from build123d import *

# Parameters (mm, degrees)
AUFSATZ_LINEAR_AUSTRAGEN1_DEPTH = 24
VERRUNDUNG1_R                   = 2
SKIZZE6_R                       = 2.3
SCHNITT_LINEAR_AUSTRAGEN2_DEPTH = 100
SKIZZE7_W                       = 12.2
SKIZZE7_H                       = 11.3
SCHNITT_LINEAR_AUSTRAGEN3_DEPTH = 56.3
SCHNITT_LINEAR_AUSTRAGEN4_DEPTH = 25
SCHNITT_LINEAR_AUSTRAGEN5_DEPTH = 13.7
VERRUNDUNG2_R                   = 2
SCHNITT_LINEAR_AUSTRAGEN6_DEPTH = 23.5


with BuildPart() as part:
    # Skizze1 → Aufsatz-Linear austragen1 (new body)
    with BuildSketch(Plane(origin=(0, 0, 0), x_dir=(1, 0, 0), z_dir=(0, 1, 0))):
        with BuildLine():
            Line((-29.15, 22), (-29.15, 0))
            Line((-29.15, 0), (-21.15, 0))
            ThreePointArc((-21.15, 0), (-17.325065737, 12.131141629), (-7.233726031, 19.87449893))
            ThreePointArc((-7.233726031, 19.87449893), (-3.065111361, 19.529851295), (-0.617075906, 16.138206757))
            ThreePointArc((-0.617075906, 16.138206757), (11.199480437, 11.635898674), (16.15, 0))
            Line((16.15, 0), (26.15, 0))
            Line((26.15, 0), (26.15, 22.8))
            Line((26.15, 22.8), (17.65, 22.8))
            Line((17.65, 22.8), (17.65, 35))
            Line((17.65, 35), (-17.45, 35))
            Line((-17.45, 35), (-17.45, 22))
            Line((-17.45, 22), (-29.15, 22))
        make_face()
    extrude(amount=AUFSATZ_LINEAR_AUSTRAGEN1_DEPTH)

    # Verrundung1
    verrundung1_edges = [part.edges().sort_by_distance(p)[0] for p in [
        (-17.45, 12, -22),
    ]]
    fillet(verrundung1_edges, radius=VERRUNDUNG1_R)

    # Skizze6 → Schnitt-Linear austragen2 (cut)
    with BuildSketch(Plane.XY):
        with Locations((-24.15, 19)):
            Circle(SKIZZE6_R)
        with Locations((-24.15, 5)):
            Circle(SKIZZE6_R)
        with BuildLine():
            Line((-25.3, 17.008141571), (-24.15, 16.344188762))
            Line((-24.15, 16.344188762), (-23, 17.008141571))
            ThreePointArc((-23, 17.008141571), (-24.15, 16.7), (-25.3, 17.008141571))
        make_face()
        with BuildLine():
            Line((-25.3, 3.008141571), (-24.15, 2.344188762))
            Line((-24.15, 2.344188762), (-23, 3.008141571))
            ThreePointArc((-23, 3.008141571), (-24.15, 2.7), (-25.3, 3.008141571))
        make_face()
    extrude(amount=-SCHNITT_LINEAR_AUSTRAGEN2_DEPTH, mode=Mode.SUBTRACT)

    # Skizze7 → Schnitt-Linear austragen3 (cut, through all)
    with BuildSketch(Plane(origin=(26.15, 0, 0), x_dir=(0, 0, -1), z_dir=(1, 0, 0))):
        with Locations((28.9, 5.65)):
            Rectangle(SKIZZE7_W, SKIZZE7_H)
    extrude(amount=-SCHNITT_LINEAR_AUSTRAGEN3_DEPTH, mode=Mode.SUBTRACT)

    # Skizze8 → Schnitt-Linear austragen4 (cut)
    with BuildSketch(Plane(origin=(0, 0, -22.8), x_dir=(-1, 0, 0), z_dir=(0, 0, -1))):
        with BuildLine():
            Line((-22.275, 3.551442841), (-21.15, 2.901923789))
            Line((-21.15, 2.901923789), (-20.025, 3.551442841))
            ThreePointArc((-20.025, 3.551442841), (-21.15, 7.75), (-22.275, 3.551442841))
        make_face()
        with BuildLine():
            Line((-22.275, 17.051442841), (-21.15, 16.401923789))
            Line((-21.15, 16.401923789), (-20.025, 17.051442841))
            ThreePointArc((-20.025, 17.051442841), (-21.15, 21.25), (-22.275, 17.051442841))
        make_face()
    extrude(amount=-SCHNITT_LINEAR_AUSTRAGEN4_DEPTH, mode=Mode.SUBTRACT)

    # Skizze10 → Schnitt-Linear austragen5 (cut, through all)
    with BuildSketch(Plane.XZ.offset(-11.3)):
        with BuildLine():
            Line((-11.45, -26.25), (12.05, -26.25))
            ThreePointArc((12.05, -26.25), (14.3, -28.5), (12.05, -30.75))
            Line((12.05, -30.75), (-11.45, -30.75))
            ThreePointArc((-11.45, -30.75), (-13.7, -28.5), (-11.45, -26.25))
        make_face()
    extrude(amount=-SCHNITT_LINEAR_AUSTRAGEN5_DEPTH, mode=Mode.SUBTRACT)

    # Verrundung2
    verrundung2_edges = [part.edges().sort_by_distance(p)[0] for p in [
        (-3.065111361, 24, -19.529851295),
        (-29.15, 0, -11),
        (11.199480437, 24, -11.635898674),
        (26.15, 0, -11.4),
        (11.199480437, 0, -11.635898674),
        (-3.065111361, 0, -19.529851295),
        (-17.325065737, 0, -12.131141629),
        (-0.617075906, 12, -16.138206757),
        (26.15, 24, -11.4),
        (21.9, 24, -22.8),
        (17.65, 24, -28.9),
        (-17.45, 24, -29.5),
        (-18.035786438, 24, -22.585786438),
        (-24.3, 24, -22),
        (-29.15, 24, -11),
        (-17.325065737, 24, -12.131141629),
        (-17.552633404, 11.3, -23.367544468),
        (17.65, 11.3, -28.9),
        (-17.45, 11.3, -29.5),
    ]]
    fillet(verrundung2_edges, radius=VERRUNDUNG2_R)

    # Skizze12 → Schnitt-Linear austragen6 (cut)
    with BuildSketch(Plane(origin=(-11.45, 0, 0), x_dir=(0, 0, -1), z_dir=(1, 0, 0))):
        Polygon((24.9, 24), (24.9, 20), (26.25, 19.220577137), (30.75, 19.220577137), (32.1, 20), (32.1, 24), align=None)
    extrude(amount=SCHNITT_LINEAR_AUSTRAGEN6_DEPTH, mode=Mode.SUBTRACT)

    # Skizze12<3> one side → Schnitt-Rotation1 (revolve, cut)
    with BuildSketch(Plane(origin=(-11.45, 0, 0), x_dir=(0, 0, -1), z_dir=(1, 0, 0))):
        Polygon((32.1, 24), (28.5, 24), (28.5, 19.220577137), (30.75, 19.220577137), (32.1, 20), align=None)
    schnitt_rotation1 = revolve(axis=Axis((-11.45, 24, -28.5), (0, -1, 0)), mode=Mode.SUBTRACT)

    # Spiegeln1: Schnitt-Rotation1 across plane
    add(schnitt_rotation1.mirror(Plane.ZY.offset(-0.3)), mode=Mode.SUBTRACT)


solid = part.part
Geometry: final body of the model. Coordinates: model frame, mm. A direction names the side the tool comes from. Give positions to 0.01 mm unless a question says otherwise; leave off trailing zeros. Answer in a Markdown table with one row per item.
(1) Draft query along Z for faces 1 (the flat face through (2, 24, -19)), 2 (the cylindrical face through (11.56, 11.86, -11.28)), 3 (the cylindrical face through (-24.37, 23.4, -21.43)), 4 (the flat face through (0.136, 19.616, -25.566)). Return one class per face: +Z half, -Z half, draft (parallel to the pull), parting line (faces both ways), or undercut.
Answers below:
| item | result |
|---|---|
| face 1 | draft |
| face 2 | +Z half |
| face 3 | -Z half |
| face 4 | undercut |
(2) Pin query (flat end, axial travel): pin 1 (5 mm diameter, centred on x = -23.5, y = 12.5, fed in from -Z); pin 2 (2.5 mm diameter, centred on y = 18, z = -30.5, fed in from +X); pin 3 (7 mm diameter, centred on y = 16, z = -28.5, fed in from -X). Return the tip coordinate at first contact, or that it passes through.
Answers below:
| item | result |
|---|---|
| pin 1 | z = -22 |
| pin 2 | x = 17.65 |
| pin 3 | x = -17.45 |
(3) Section query A-A on z = -19. State how many separate pieces and enclosed holes the cut face has, then the cut area to 3 significant figures.
Answers below:
| item | result |
|---|---|
| separate pieces | 2 |
| enclosed holes | 4 |
| area | 1,080 mm^2 |
(4) Set-up query: faces 5 (the cylindrical face through (17.05, 23.43, -28)), 6 (the flat face through (17.65, 18, -29)), 7 (the flat face through (21.72, 3.23, -11.56)), 8 (the cylindrical face through (15.65, 22.03, -28.42)). Return all of +Z, -Z, +X, -X, +Y, -Y with unobstructed straight access to the full face (end or side cutting, diameter ignored); none if empty.
Answers below:
| item | result |
|---|---|
| face 5 | -Z, +X, +Y |
| face 6 | -Z, +X, +Y, -Y |
| face 7 | +Z, -Z |
| face 8 | +Y |
(5) Ray query, line 1 along Y through (x, z) = (21.15, -12); line 2 along Y through (x, z) = (21, -3) (3 decimals); line 3 along X through (y, z) = (5, -9). Return the intervals inside material, ascending. Write a range as [from, to].
Answers below:
| item | result |
|---|---|
| line 1 | [0, 2.9], [7.75, 16.4], [21.25, 24] |
| line 2 | [0, 2.989], [7.745, 16.489], [21.245, 24] |
| line 3 | [-29.15, -26.45], [-21.85, -19.14], [13.41, 18.96], [23.34, 26.15] |
